from build123d import *

# Parameters (mm, degrees)
BOSS_EXTRUDE1_DEPTH = 5
SKETCH2_OUTSIDE_W   = 60.516
SKETCH2_OUTSIDE_H   = 58.796
SKETCH2_OUTSIDE_R   = 8.199202844
CUT_EXTRUDE1_DEPTH  = 10
CUT_EXTRUDE1_TAPER  = 60
SKETCH3_OUTSIDE_W   = 29.34
SKETCH3_OUTSIDE_H   = 27.62
SKETCH3_OUTSIDE_R   = 8.172152793
CUT_EXTRUDE2_DEPTH  = 1
CUT_EXTRUDE2_TAPER  = 60
SKETCH4_R           = 5
CUT_EXTRUDE3_DEPTH  = 8


with BuildPart() as part:
    # Sketch1 → Boss-Extrude1 (new body)
    with BuildSketch(Plane.XY):
        Polygon((9.359699903, 0), (4.68, 8.5), (-4.68, 8.5), (-9.36, -0.105997779), (-4.68, -8.5), (4.68, -8.5), align=None)
    extrude(amount=BOSS_EXTRUDE1_DEPTH)

    # Sketch2 outside → Cut-Extrude1 (cut)
    with BuildSketch(Plane.XY.offset(5)):
        Rectangle(SKETCH2_OUTSIDE_W, SKETCH2_OUTSIDE_H)
        Circle(SKETCH2_OUTSIDE_R, mode=Mode.SUBTRACT)
    extrude(amount=-CUT_EXTRUDE1_DEPTH, taper=CUT_EXTRUDE1_TAPER, mode=Mode.SUBTRACT)

    # Sketch3 outside → Cut-Extrude2 (cut)
    with BuildSketch(Plane(origin=(0, 0, 0), x_dir=(-1, 0, 0), z_dir=(0, 0, -1))):
        Rectangle(SKETCH3_OUTSIDE_W, SKETCH3_OUTSIDE_H)
        Circle(SKETCH3_OUTSIDE_R, mode=Mode.SUBTRACT)
    extrude(amount=-CUT_EXTRUDE2_DEPTH, taper=CUT_EXTRUDE2_TAPER, mode=Mode.SUBTRACT)

    # Sketch4 → Cut-Extrude3 (cut)
    with BuildSketch(Plane.XY.offset(5)):
        Circle(SKETCH4_R)
    extrude(amount=-CUT_EXTRUDE3_DEPTH, mode=Mode.SUBTRACT)


solid = part.part
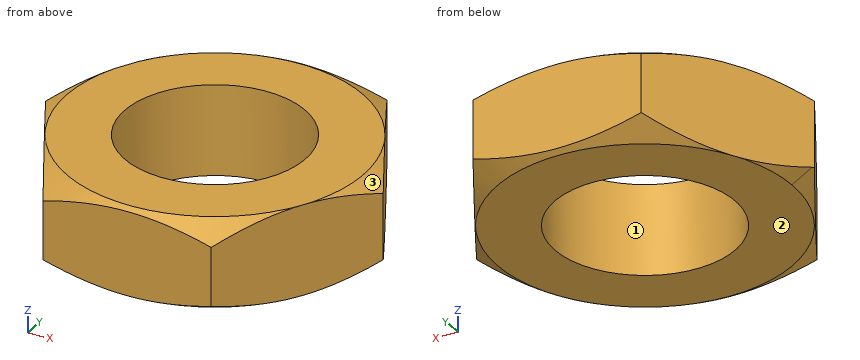
Part model, mm, in its own coordinate system. Face numbers are marked on the shaded views. Round coordinates to 2 decimals unless told otherwise and drop trailing zeros. Write each loop counter-clockwise with the first axis right and the second up, starting at its lowest first coordinate (ties: lowest second). Pieces come first, ordered by that corner, then holes. Notation, with made-up numbers: M 62,12 L 92,12 A23 ccw 92,24 Z; hole C 61,23.25 d3. An arc over 180 degrees is marked long. Return JSON: item names as keys, results as strings. Group by question number.
(1) Drill centre lines: probe 1 along Y at (x, z) = (0, 1.1); probe 2 along X at (y, z) = (-1, 1.05); probe 3 along Y at (x, z) = (-4.25, 1.9). Where is each one in solid material? Low to high.
(2) Two-plate mould, pull along X, no slides. Class the marked faces 1, 2 and 3: +X half, -X half, draft (parallel to the pull), parting line (faces both ways), or undercut.
(3) Pin check, flat tip, straight feed: pin 1 Ø1.5 at (x, z) = (-5.5, 3) entering from -Y. Stop position of the tip, or through.
(4) Saw through at A-A on x = 0. Write the cut outline in (y, z).
(5) Saw through at B-B on z = 3.25. Write the cut outline in (x, y), then the cut area to 3 significant figures.
Returned:
{
 "1": {"probe 1": "-8.5 to -5, 5 to 8.5", "probe 2": "-8.86 to -4.9, 4.9 to 8.81", "probe 3": "-8.5 to -2.63, 2.63 to 8.5"},
 "2": {"face 1": "undercut", "face 2": "draft", "face 3": "+X half"},
 "3": {"pin 1": "y = -8.37"},
 "4": {"outline": "M -8.5,0.19 L -8.17,0 L -5,0 L -5,5 L -8.2,5 L -8.5,4.83 Z; M 5,0 L 8.17,0 L 8.5,0.19 L 8.5,4.83 L 8.2,5 L 5,5 Z"},
 "5": {"outline": "M -9.36,-0.11 L -4.68,-8.5 L 4.68,-8.5 L 9.36,0 L 4.68,8.5 L -4.68,8.5 Z; hole C 0,0 d10", "area": "160 mm²"}
}
